Design review of the part built by this model. Coordinates are the model's own, in mm. Face numbers are marked on the shaded views. A direction names the side the tool comes from. Round coordinates to 2 decimals unless told otherwise and drop trailing zeros. Loops run counter-clockwise (first coordinate to the right, second up) from the corner with the lowest first, then second, coordinate; pieces in that order, holes last. Notation, with made-up numbers: (-33, 58.5) - (-19, 58.5) arc R12 ccw to (-19, 70.5) - close; hole circle Ø3 at (-26.5, -26.5). An arc over 180 degrees is marked (long way). Return JSON: item names as keys, results as strings. Group by question number.
from build123d import *

# Parameters (mm, degrees)
SKETCH1_W                = 25
SKETCH1_H                = 6.75
BOSS_EXTRUDE1_DEPTH      = 6.5
BOSS_EXTRUDE4_DEPTH      = 6.5
BOSS_EXTRUDE3_DEPTH      = 6
BOSS_EXTRUDE3_DEPTH_BACK = 4.95
SKETCH4_W                = 2.3
SKETCH4_H                = 4.5
CUT_EXTRUDE1_DEPTH       = 23
SKETCH6_R                = 2.55
CUT_EXTRUDE2_DEPTH       = 10
BOSS_EXTRUDE5_DEPTH      = 1.575
CUT_EXTRUDE3_DEPTH       = 3
SKETCH9_R                = 0.8
CUT_EXTRUDE4_DEPTH       = 10.95
BOSS_EXTRUDE6_DEPTH      = 0.25


with BuildPart() as part:
    # Sketch1 → Boss-Extrude1 (new body)
    with BuildSketch(Plane(origin=(0, 0, 0), x_dir=(1, 0, 0), z_dir=(0, 1, 0))):
        with Locations((12.5, -3.375)):
            Rectangle(SKETCH1_W, SKETCH1_H)
    extrude(amount=BOSS_EXTRUDE1_DEPTH)

    # Sketch5 → Boss-Extrude4 (add)
    with BuildSketch(Plane(origin=(0, 6.5, 0), x_dir=(1, 0, 0), z_dir=(0, 1, 0))):
        Polygon((-5.715767665, -3.375), (-2.857883832, -8.325), (2.857883832, -8.325), (5.715767665, -3.375), (2.857883832, 1.575), (-2.857883832, 1.575), align=None)
    extrude(amount=-BOSS_EXTRUDE4_DEPTH)

    # Sketch3 → Boss-Extrude3 (add, two sides)
    with BuildSketch(Plane.XY.offset(3.375)) as boss_extrude3_sk:
        Polygon((21.602997682, 14.262034616), (26.527036447, 15.130275504), (30, -4.565879556), (25.075961235, -5.434120444), align=None)
    extrude(amount=BOSS_EXTRUDE3_DEPTH)
    extrude(boss_extrude3_sk.sketch, amount=-BOSS_EXTRUDE3_DEPTH_BACK)

    # Sketch4 → Cut-Extrude1 (cut)
    with BuildSketch(Plane(origin=(-1.787541475, 10.137651469, 0), x_dir=(0.984807753, 0.173648178, 0), z_dir=(-0.173648178, 0.984807753, 0))):
        with Locations((27.601375926, -2.675)):
            Rectangle(SKETCH4_W, SKETCH4_H)
    extrude(amount=-CUT_EXTRUDE1_DEPTH, mode=Mode.SUBTRACT)

    # Sketch6 → Cut-Extrude2 (cut)
    with BuildSketch(Plane(origin=(0, 6.5, 0), x_dir=(1, 0, 0), z_dir=(0, 1, 0))):
        with Locations((0, -3.335615973)):
            Circle(SKETCH6_R)
    extrude(amount=-CUT_EXTRUDE2_DEPTH, mode=Mode.SUBTRACT)

    # Sketch7 → Boss-Extrude5 (add)
    with BuildSketch(Plane(origin=(0, 0, -1.575), x_dir=(-1, 0, 0), z_dir=(0, 0, -1))):
        Polygon((-2.857883832, 0), (-24.117779184, 0), (-25.075961235, -5.434120444), (-30, -4.565879556), (-26.527036447, 15.130275504), (-21.602997682, 14.262034616), (-22.97165381, 6.5), (-2.857883832, 6.5), align=None)
    extrude(amount=-BOSS_EXTRUDE5_DEPTH)

    # Sketch8 → Cut-Extrude3 (cut)
    with BuildSketch(Plane(origin=(0, 0, 0), x_dir=(-1, 0, 0), z_dir=(0, -1, 0))):
        Polygon((-4.67653718, -11.475), (4.67653718, -11.475), (9.353074361, -3.375), (4.67653718, 4.725), (-4.67653718, 4.725), (-9.353074361, -3.375), align=None)
    extrude(amount=-CUT_EXTRUDE3_DEPTH, mode=Mode.SUBTRACT)

    # Sketch9 → Cut-Extrude4 (cut)
    with BuildSketch(Plane(origin=(0, 0, -1.575), x_dir=(-1, 0, 0), z_dir=(0, 0, -1))):
        with Locations((-28.459277655, -3.314410557)):
            Circle(SKETCH9_R)
        with Locations((-27.591036766, 1.609628208)):
            Circle(SKETCH9_R)
        with Locations((-26.722795878, 6.533666973)):
            Circle(SKETCH9_R)
        with Locations((-25.85455499, 11.457705738)):
            Circle(SKETCH9_R)
    extrude(amount=-CUT_EXTRUDE4_DEPTH, mode=Mode.SUBTRACT)

    # Sketch10 → Boss-Extrude6 (add)
    with BuildSketch(Plane.XY.offset(6.75)):
        Polygon((11.821517388, 5.121255448), (12.792571074, 5.121255448), (12.792571074, 1.621255448), (12.164365946, 1.621255448), (12.164365946, 4.537922115), (11.446417228, 4.537922115), align=None)
        with BuildLine():
            add(Edge.make_bspline(
                [(15.048079888, 5.210999038), (15.078487624, 5.210547627), (15.138277356, 5.209660031), (15.226336378, 5.20004665), (15.311161562, 5.185523511), (15.393084756, 5.165268798), (15.471516268, 5.138462406), (15.54702694, 5.106375614), (15.618717974, 5.067325404), (15.687503662, 5.023216186), (15.753357507, 4.973278299), (15.814696757, 4.916346529), (15.872641599, 4.853730878), (15.925937739, 4.784484711), (15.975765436, 4.709237895), (16.021960966, 4.627978498), (16.064170689, 4.540308809), (16.102867677, 4.446070622), (16.137470646, 4.343851347), (16.166616684, 4.232478485), (16.191614288, 4.111926601), (16.21271403, 3.981895624), (16.228662025, 3.842212712), (16.239411294, 3.692970662), (16.246787952, 3.534457192), (16.247389983, 3.425718255), (16.247699279, 3.369853205)],
                knots=[0, 0, 0, 0, 9.1189e-05, 0.000179302, 0.000265406, 0.000349239, 0.000432161, 0.00051382, 0.000595069, 0.000676752, 0.000758786, 0.000842642, 0.00092749, 0.00101444, 0.001104474, 0.001198046, 0.001294628, 0.001396185, 0.001503495, 0.001618119, 0.001741326, 0.001872727, 0.002013179, 0.002162939, 0.002321548, 0.002489129, 0.002489129, 0.002489129, 0.002489129], degree=3))
            add(Edge.make_bspline(
                [(16.247699279, 3.369853205), (16.247365014, 3.31328922), (16.246715542, 3.203386413), (16.239717944, 3.043423099), (16.22766775, 2.893097462), (16.212136589, 2.752425056), (16.190863148, 2.621480168), (16.165948991, 2.499923737), (16.136342892, 2.387799826), (16.100600112, 2.285361073), (16.062137358, 2.190957383), (16.019812173, 2.10345863), (15.974362278, 2.022627817), (15.926830158, 1.947245503), (15.874609927, 1.87953392), (15.82024329, 1.817190519), (15.761363027, 1.762590042), (15.700448226, 1.712918623), (15.635267329, 1.66999255), (15.566492532, 1.632450114), (15.492897697, 1.601998739), (15.415824335, 1.57551376), (15.333958715, 1.556500403), (15.248601668, 1.541413929), (15.158789533, 1.533076218), (15.097641814, 1.53204187), (15.066309055, 1.531511859)],
                knots=[0, 0, 0, 0, 0.000169685, 0.000329694, 0.000480207, 0.000622052, 0.000754146, 0.000878038, 0.000994198, 0.001101735, 0.001203292, 0.001299874, 0.001393102, 0.001481398, 0.001566938, 0.001649385, 0.001729242, 0.001807533, 0.001884926, 0.001963041, 0.002042215, 0.002123584, 0.00220725, 0.002294045, 0.002383484, 0.002477476, 0.002477476, 0.002477476, 0.002477476], degree=3))
            add(Edge.make_bspline(
                [(15.066309055, 1.531511859), (15.034977142, 1.532052093), (14.973598385, 1.533110405), (14.883543389, 1.541351934), (14.797733993, 1.556561518), (14.715220684, 1.575659731), (14.63657774, 1.601940139), (14.561428072, 1.633302597), (14.490349515, 1.670610787), (14.423145264, 1.713636874), (14.360044773, 1.762975953), (14.300067462, 1.818100286), (14.243346003, 1.878870149), (14.19074327, 1.945966213), (14.141397784, 2.018492887), (14.095824138, 2.097278389), (14.054049723, 2.18220801), (14.014767826, 2.273400132), (13.980636829, 2.372818019), (13.950261828, 2.481349457), (13.925379425, 2.599899148), (13.905367332, 2.728429006), (13.889389688, 2.866666733), (13.877504158, 3.014679055), (13.870467691, 3.17253491), (13.869825031, 3.281037103), (13.869494151, 3.33690048)],
                knots=[0, 0, 0, 0, 9.3992e-05, 0.000184129, 0.000270924, 0.000355272, 0.000437971, 0.000519356, 0.000599327, 0.000678482, 0.000758422, 0.000839307, 0.000922649, 0.001007511, 0.001094825, 0.001185617, 0.00128031, 0.001378632, 0.00148329, 0.001595393, 0.001716541, 0.001846447, 0.001985506, 0.002133922, 0.00229183, 0.002459412, 0.002459412, 0.002459412, 0.002459412], degree=3))
            add(Edge.make_bspline(
                [(13.869494151, 3.33690048), (13.870093509, 3.414518246), (13.871249978, 3.564282724), (13.885905598, 3.78064885), (13.907416331, 3.980641854), (13.939010504, 4.163927197), (13.978076261, 4.331183713), (14.028101996, 4.481309605), (14.085052658, 4.6163822), (14.133581938, 4.696400019), (14.156954087, 4.734937339)],
                knots=[0, 0, 0, 0, 0.00023281, 0.000449211, 0.000650286, 0.000835979, 0.001006883, 0.001164965, 0.001310334, 0.001445389, 0.001445389, 0.001445389, 0.001445389], degree=3))
            add(Edge.make_bspline(
                [(14.156954087, 4.734937339), (14.184130109, 4.772796391), (14.237264587, 4.846818296), (14.330171707, 4.943995222), (14.42998831, 5.027105688), (14.538764575, 5.094268828), (14.654780157, 5.147233687), (14.77903111, 5.18464217), (14.911058597, 5.206438095), (15.001724074, 5.209456021), (15.048079888, 5.210999038)],
                knots=[0, 0, 0, 0, 0.000139664, 0.000273071, 0.000402072, 0.00052834, 0.000655415, 0.000783615, 0.000916514, 0.00105555, 0.00105555, 0.00105555, 0.00105555], degree=3))
        make_face()
        with BuildLine():
            add(Edge.make_bspline(
                [(15.063504568, 4.58279391), (15.036015723, 4.581490993), (14.982122994, 4.578936585), (14.903922078, 4.557253264), (14.830183496, 4.523762204), (14.774092526, 4.483460951), (14.732108993, 4.444827367), (14.702774798, 4.409865229), (14.674486589, 4.370850003), (14.649501019, 4.326021133), (14.625908119, 4.276989372), (14.602850744, 4.223532146), (14.583949751, 4.16433643), (14.565380027, 4.100410333), (14.549111215, 4.029986471), (14.535481518, 3.952489204), (14.523304581, 3.867414562), (14.514811023, 3.77470682), (14.506892478, 3.674462974), (14.501216089, 3.566459719), (14.498842934, 3.450726192), (14.49808858, 3.371022229), (14.497699279, 3.329889262)],
                knots=[0, 0, 0, 0, 8.233e-05, 0.000161411, 0.000241719, 0.000324202, 0.000367359, 0.000412607, 0.000460858, 0.000511731, 0.000566293, 0.000624109, 0.000686189, 0.000752544, 0.000823804, 0.000902881, 0.00098855, 0.001081546, 0.001182103, 0.001290221, 0.00140594, 0.001529346, 0.001529346, 0.001529346, 0.001529346], degree=3))
            add(Edge.make_bspline(
                [(14.497699279, 3.329889262), (14.498340021, 3.276599515), (14.499568691, 3.174412475), (14.50600389, 3.027463952), (14.518902713, 2.893728963), (14.534946244, 2.772301138), (14.557480038, 2.663967967), (14.583406627, 2.567704519), (14.61542366, 2.484737918), (14.65242551, 2.413868282), (14.693406726, 2.35357963), (14.737893638, 2.302334004), (14.784371628, 2.257957709), (14.834291423, 2.221911392), (14.887533931, 2.194287156), (14.943654674, 2.174417385), (15.002689316, 2.16225427), (15.043115631, 2.160567637), (15.063504568, 2.159716987)],
                knots=[0, 0, 0, 0, 0.00015988, 0.000306582, 0.00044109, 0.000562851, 0.000673817, 0.000772822, 0.000861618, 0.000940022, 0.001012169, 0.001079776, 0.001143265, 0.001204556, 0.001263825, 0.001322589, 0.001382678, 0.00144382, 0.00144382, 0.00144382, 0.00144382], degree=3))
            add(Edge.make_bspline(
                [(15.063504568, 2.159716987), (15.083193821, 2.160299065), (15.121742931, 2.161438701), (15.177956166, 2.173136917), (15.231115396, 2.192155675), (15.281060116, 2.219059043), (15.327968971, 2.253270793), (15.3716127, 2.294941264), (15.411662151, 2.344485814), (15.434995142, 2.381255198), (15.447018189, 2.400201762)],
                knots=[0, 0, 0, 0, 5.8998e-05, 0.000115512, 0.000171399, 0.00022786, 0.000285078, 0.000345085, 0.000408376, 0.000475658, 0.000475658, 0.000475658, 0.000475658], degree=3))
            add(Edge.make_bspline(
                [(15.447018189, 2.400201762), (15.461173303, 2.426091637), (15.490855427, 2.480380606), (15.525203632, 2.571991216), (15.554116037, 2.675312843), (15.579000521, 2.790667033), (15.596019991, 2.918508758), (15.610677137, 3.058027363), (15.617746642, 3.209925406), (15.618896536, 3.315160919), (15.619494151, 3.369853205)],
                knots=[0, 0, 0, 0, 8.843e-05, 0.000185431, 0.00029262, 0.000410194, 0.000539093, 0.000679319, 0.000830958, 0.000995045, 0.000995045, 0.000995045, 0.000995045], degree=3))
            add(Edge.make_bspline(
                [(15.619494151, 3.369853205), (15.619263305, 3.425020246), (15.618818967, 3.531207384), (15.61066664, 3.683651511), (15.599313902, 3.822883921), (15.582708123, 3.948593764), (15.561341771, 4.061086209), (15.535007661, 4.160353902), (15.503961704, 4.246592481), (15.467144899, 4.319715953), (15.426368, 4.381860874), (15.383082077, 4.435176395), (15.3371041, 4.480695842), (15.288510958, 4.518590513), (15.236177946, 4.547544883), (15.181104694, 4.567989064), (15.123178296, 4.580357108), (15.083664292, 4.581970679), (15.063504568, 4.58279391)],
                knots=[0, 0, 0, 0, 0.000165478, 0.000318517, 0.00045785, 0.000584474, 0.000698739, 0.000801125, 0.000892295, 0.000973192, 0.001046115, 0.001114882, 0.001178838, 0.00123984, 0.001299154, 0.001357499, 0.001415527, 0.00147597, 0.00147597, 0.00147597, 0.00147597], degree=3))
        make_face(mode=Mode.SUBTRACT)
        Polygon((17.234878766, 5.210999038), (17.8182121, 5.210999038), (17.672378766, 4.537922115), (18.215748157, 5.013983814), (18.491289023, 4.537922115), (17.773340305, 4.335999038), (18.491289023, 4.134075961), (18.180692068, 3.647497435), (17.6541496, 4.134075961), (17.8182121, 3.460999038), (17.234878766, 3.460999038), (17.412262581, 4.134075961), (16.873801042, 3.647497435), (16.561801843, 4.134075961), (17.279750561, 4.335999038), (16.561801843, 4.537922115), (16.873801042, 5.036419711), (17.412262581, 4.537922115), align=None)
    extrude(amount=BOSS_EXTRUDE6_DEPTH)


solid = part.part
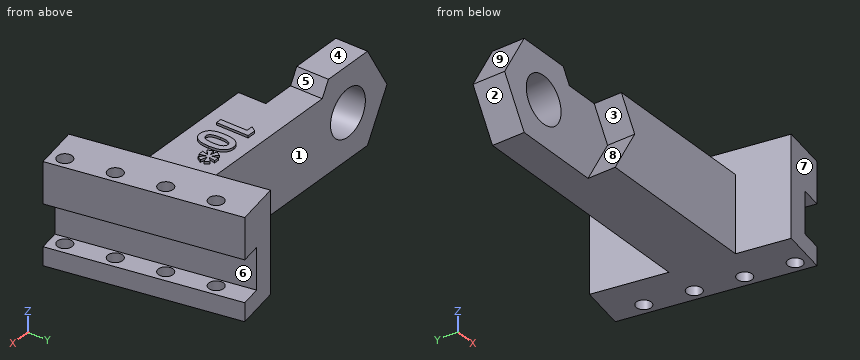
Q1. Add section A-A, the plane x = 0. State the section outline as (y, z) points (3 decimals).
Q2. Insertion check: pin 1 Ø1.4 at (x, y) = (28.46, -3.31) entering from -Z; pin 2 Ø1.5 at (y, z) = (3, 7.5) entering from +X; pin 3 Ø3 at (x, y) = (1, 5) entering from +Z (3 decimals). Each pin has a flat end and moves straight along its axis. Give the tip position at first contact, or say it passes through.
Q3. Add section D-D, the plane y = 7.75. State the section outline as (x, z) points (3 decimals), plus the area to 3 significant figures.
Q4. Add section B-B, the plane z = 6.25. State the section outline as (x, y) points, plus the area to 3 significant figures.
Q5. Tool access review of the marked faces 5, 6, 7, 8 and 9: name each direction out of +Z, -Z, +X, -X, +Y, -Y from which nothing blocks a thin tool from reaching the whole face with its end or side.
Q6. Draft analysis for pull direction Z (two halves, no side actions). For the marked faces 1, 2, 3 and 4, state which applies: pulls with the +Z half, pulls with the -Z half, needs draft (parallel to the pull), parting line crosses it, or undercut.
Q7. Add section C-C, the plane z = 1.5. State the section outline as (x, y) points, plus the area to 3 significant figures.
Q8. For line 1 (Y direction, x = 12.5, z = 5.25); line 2 (Z direction, x = 0, y = 3.95) (3 decimals); line 3 (Z direction, x = 4, y = 5.75) (3 decimals), list the stretches that pass through material, from the lowest coordinate up.
Evaluation:
{
 "1": {"outline": "(3, -1.575) - (6.5, -1.575) - (6.5, 0.786) - (3, 0.786) - close; (3, 5.886) - (6.5, 5.886) - (6.5, 8.325) - (3, 8.325) - close"},
 "2": {"pin 1": "through", "pin 2": "x = 28.8", "pin 3": "z = 8.325"},
 "3": {"outline": "(22.751, -1.575) - (27.828, -1.575) - (27.828, 0.425) - (25.493, 0.425) - (25.493, 4.925) - (27.828, 4.925) - (27.828, 9.375) - (22.751, 9.375) - close", "area": "45.1 mm²"},
 "4": {"outline": "(-4.06, 3) - (7.69, 3) - (7.69, 0) - (24.12, 0) - (25.08, -5.43) - (30, -4.57) - (26.53, 15.13) - (21.6, 14.26) - (22.97, 6.5) - (-4.06, 6.5) - close; hole circle Ø1.6 at (25.85, 11.46); hole circle Ø1.6 at (26.72, 6.53); hole circle Ø1.6 at (27.59, 1.61); hole circle Ø1.6 at (28.46, -3.31)", "area": "236 mm²"},
 "5": {"face 5": "+Z, +Y, -Y", "face 6": "+X, +Y", "face 7": "+Z, -Z, +X, -Y", "face 8": "-X, -Y", "face 9": "+Z, -X, +Y, -Y"},
 "6": {"face 1": "needs draft", "face 2": "pulls with the -Z half", "face 3": "undercut", "face 4": "pulls with the +Z half"},
 "7": {"outline": "(-4.63, 3) - (-1.77, 3) - (-1.77, 6.5) - (-4.63, 6.5) - close; (1.77, 3) - (8.27, 3) - (8.27, 0) - (24.12, 0) - (25.08, -5.43) - (27.73, -4.97) - (24.26, 14.73) - (21.6, 14.26) - (22.97, 6.5) - (1.77, 6.5) - close", "area": "186 mm²"},
 "8": {"line 1": "0 to 6.5", "line 2": "-1.575 to 0.786, 5.886 to 8.325", "line 3": "-1.575 to 6.75"}
}
